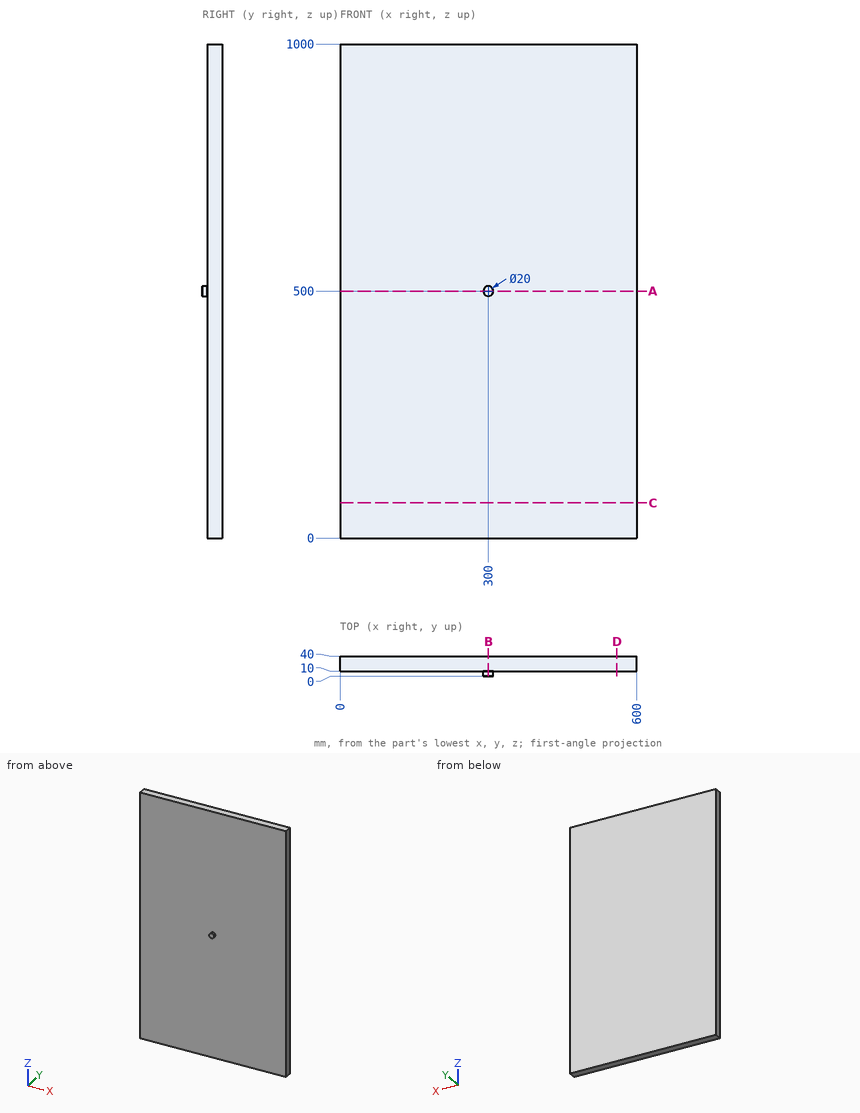
Print and shaded views of the part. All mm, measured from the part's lowest x, y and z. Round coordinates to 2 decimals unless told otherwise and drop trailing zeros. Write each loop counter-clockwise with the first axis right and the second up, starting at its lowest first coordinate (ties: lowest second). Pieces come first, ordered by that corner, then holes. Notation, with made-up numbers: (12, 7) - (63, 7) arc R11 cw to (63, 17) - close; hole circle Ø10 at (24.5, 57). An arc over 180 degrees is marked (long way). One line per item, written item: value.
(1) Cut at C-C, the plane z = 71.5. Give the cut face in (x, y), plus the area to 3 significant figures.
Values follow:
outline: (0, 10) - (600, 10) - (600, 40) - (0, 40) - close
area: 18,000 mm²
(2) Cut at A-A, the plane z = 500. Give the cut face in (x, y), plus the area to 3 significant figures.
Values follow:
outline: (0, 10) - (290, 10) - (290, 0) - (310, 0) - (310, 10) - (600, 10) - (600, 40) - (0, 40) - close
area: 18,200 mm²
(3) Cut at D-D, the plane x = 560. Give the cut face in (y, z).
Values follow:
outline: (10, 0) - (40, 0) - (40, 1000) - (10, 1000) - close
(4) Cut at B-B, the plane x = 300. Give the cut face in (y, z).
Values follow:
outline: (0, 490) - (10, 490) - (10, 0) - (40, 0) - (40, 1000) - (10, 1000) - (10, 510) - (0, 510) - close
(5) Wall check: probe 1 along Y at (x, z) = (438, 327.5). Give the ranges that are in metal, low to high.
Values follow:
probe 1: y = 10 to 40
